Geometry check sheet. Reference: the model listing, model coordinates, mm. A direction names the side the tool comes from. Give positions to 0.01 mm unless a question says otherwise; leave off trailing zeros. Write each loop counter-clockwise with the first axis right and the second up, starting at its lowest first coordinate (ties: lowest second). Pieces come first, ordered by that corner, then holes. Notation, with made-up numbers: M 43,72.5 L 62,72.5 A25 cw 62,106.5 Z; hole C -27.75,-34 d11. An arc over 180 degrees is marked long. Use one line per item in the form item = value. Start each with the question number.
```python
from build123d import *

# Parameters (mm, degrees)
SKETCH1_W           = 50
SKETCH1_H           = 30
BOSS_EXTRUDE1_DEPTH = 10
SHELL4_T            = -1
SKETCH9_W           = 2
SKETCH9_H           = 15
CUT_EXTRUDE5_DEPTH  = 63.649820431
SKETCH10_R          = 1.5
CUT_EXTRUDE6_DEPTH  = 21


with BuildPart() as part:
    # Sketch1 → Boss-Extrude1 (new body)
    with BuildSketch(Plane.XY):
        Rectangle(SKETCH1_W, SKETCH1_H)
    extrude(amount=BOSS_EXTRUDE1_DEPTH)

    # Shell4
    shell4_openings = [part.faces().sort_by_distance(p)[0] for p in [
        (0, 0, 0),
    ]]
    offset(amount=SHELL4_T, openings=shell4_openings, kind=Kind.INTERSECTION)

    # Sketch9 → Cut-Extrude5 (cut, through all)
    with BuildSketch(Plane(origin=(35, 0, 0), x_dir=(0, 0, -1), z_dir=(1, 0, 0))):
        with Locations((-3.225993387, -0.726962262)):
            Rectangle(SKETCH9_W, SKETCH9_H)
    extrude(amount=-CUT_EXTRUDE5_DEPTH, mode=Mode.SUBTRACT)

    # Sketch10 → Cut-Extrude6 (cut)
    with BuildSketch(Plane(origin=(0, 25, 0), x_dir=(1, 0, 0), z_dir=(0, 1, 0))):
        with Locations(Location((-20.534888549, -5.815355869, 0), (0, 0, 90))):
            Circle(SKETCH10_R)
    extrude(amount=-CUT_EXTRUDE6_DEPTH, mode=Mode.SUBTRACT)


solid = part.part
```
(1) Sectioned sample at A-A, the plane z = 3. Record the boundary of the cut face in (x, y).
(2) Depth check by flat-ended pin: pin 1 (2.5 mm diameter, centred on x = -20.53, z = 5.82, fed in from +Y); pin 2 (2 mm diameter, centred on y = 2.5, z = 2.5, fed in from -X); pin 3 (1 mm diameter, centred on x = -15, y = -9, fed in from -Z). Enter the tip coordinate at first touch or a pass-through.
(3) Sectioned sample at C-C, the plane x = 8. Record the boundary of the cut face in (y, z).
(4) Draft check along Z on faces 4 (the flat face through (0, 0, 9)), 5 (the flat face through (24, -0.2, 4.4)), 6 (the flat face through (24.5, -8.227, 3.2)). Enter one of: released by +Z, released by -Z, zero draft, split by the parting line, or undercut.
(5) Thickness scan on probe 1 along X at (y, z) = (5, 6); probe 2 along Y at (x, z) = (-21.5, 3.25); probe 3 along Z at (x, y) = (4, -12). Record the ranges inside material, lowest first. Write a range as [from, to].
(6) Sectioned sample at D-D, the plane y = -13. Record the boundary of the cut face in (x, z).
(7) Tool access check on faces 1 (the flat face through (0, 14, 4)), 2 (the flat face through (-24.5, -0.8, 4.226)), 3 (the cylindrical face through (-19.204, 14.507, 5.123)). Record the directions out of +Z, -Z, +X, -X, +Y, -Y that give a thin tool (end or side, any length) a straight path to the whole face; none if there is none.
(8) Sectioned sample at B-B, the plane y = 0. Record the boundary of the cut face in (x, z), plus the area to 3 significant figures.
Numbers:
q1.outline = M -25,-15 L 25,-15 L 25,-8.23 L 24,-8.23 L 24,-14 L -24,-14 L -24,-8.23 L -25,-8.23 Z; M -25,6.77 L -24,6.77 L -24,14 L 24,14 L 24,6.77 L 25,6.77 L 25,15 L -25,15 Z
q2.pin_1 = -14
q2.pin_2 = -25
q2.pin_3 = 9
q3.outline = M -15,0 L -14,0 L -14,9 L 14,9 L 14,0 L 15,0 L 15,10 L -15,10 Z
q4.face_4 = released by -Z
q4.face_5 = zero draft
q4.face_6 = undercut
q5.probe_1 = [-25, -24], [24, 25]
q5.probe_2 = [-15, -14], [14, 15]
q5.probe_3 = [9, 10]
q6.outline = M -25,0 L -24,0 L -24,9 L 24,9 L 24,0 L 25,0 L 25,10 L -25,10 Z
q7.face_1 = -Z
q7.face_2 = +X, -X
q7.face_3 = +Y
q8.outline = M -25,0 L -24,0 L -24,2.23 L -25,2.23 Z; M -25,4.23 L -24,4.23 L -24,9 L 24,9 L 24,4.23 L 25,4.23 L 25,10 L -25,10 Z; M 24,0 L 25,0 L 25,2.23 L 24,2.23 Z
q8.area = 64.0 mm2
